from build123d import *

# Parameters (mm, degrees)
F1_DEPTH = 25.4
F3_D     = 7.874
F5_D     = 7.874


with BuildPart() as f1:
    # F0 (on Right) → F1 (new body, symmetric)
    with BuildSketch(Plane.YZ):
        with BuildLine():
            ThreePointArc((0, 160.2718698293), (0.8845331432, 155.615181848), (3.4149201504, 151.6071544741))
            Line((3.4149201504, 151.6071544741), (322.2393654787, -190.0440494609))
            ThreePointArc((322.2393654787, -190.0440494609), (323.4580585518, -191.9333664625), (323.9420015649, -194.1289371625))
            Line((323.9420015649, -194.1289371625), (327.3172136475, -280.67))
            Line((327.3172136475, -280.67), (336.2139723666, -280.67))
            Line((336.2139723666, -280.67), (332.7884473544, -192.8389043312))
            ThreePointArc((332.7884473544, -192.8389043312), (331.8205613281, -188.4477629311), (329.3831751819, -184.6691289279))
            Line((329.3831751819, -184.6691289279), (10.5974600752, 156.9405718319))
            ThreePointArc((10.5974600752, 156.9405718319), (9.3322665716, 158.9445855188), (8.89, 161.2729295095))
            Line((8.89, 161.2729295095), (8.89, 206.0665714286))
            Line((8.89, 206.0665714286), (0, 206.0665714286))
            Line((0, 206.0665714286), (0, 160.2718698293))
        make_face()
    extrude(amount=F1_DEPTH, both=True)

    # F3 (through all)
    with Locations(Plane(origin=(0, 8.89, 0), x_dir=(-1, 0, 0), z_dir=(0, 1, 0))):
        with Locations((0, 183.669750469)):
            Hole(F3_D / 2)

    # F5 (through all)
    with Locations(Plane(origin=(0, 315.8902243159, 12.3201225744), x_dir=(1, 0, 0), z_dir=(0, -0.9992403167, -0.0389716498))):
        with Locations((0, -227.6844431866), (0, -272.1344431866)):
            Hole(F5_D / 2)


solid = f1.part
Model file for the job. Use its own axes, mm. A direction names the side the tool comes from. Round coordinates to 2 decimals unless told otherwise and drop trailing zeros. Loops run counter-clockwise (first coordinate to the right, second up) from the corner with the lowest first, then second, coordinate; pieces in that order, holes last.
1. Drop flat-ended pins along their axis: P1, Ø2, axis at x = -19.5, y = 93.5, coming from the +Z side; P2, Ø4, axis at x = -4, z = -43.5, coming from the -Y side; P3, Ø10, axis at x = -3, z = -193.5, coming from the +Y side. Give the stop position or say it passes through.
Check values:
P1: stops at z = 69.17
P2: stops at y = 183.62
P3: stops at y = 333.01
2. Band-saw the part on B-B, the plane y = 33.5. List the corners of the cut face in (x, z).
Check values:
outline: (-25.4, 119.37) - (25.4, 119.37) - (25.4, 132.4) - (-25.4, 132.4) - close
3. Wall check: probe 1 along Z at (x, y) = (0, 3.5); probe 2 along Z at (x, y) = (0, 2); probe 3 along Y at (x, z) = (17, 79). Give the ranges that are in metal, low to high.
Check values:
probe 1: z = 151.52 to 179.73, 187.61 to 206.07
probe 2: z = 153.43 to 179.73, 187.61 to 206.07
probe 3: y = 71.17 to 83.33
4. Tool access for faces 1 (the flat face through (0.36, 160.6, -16.83)), 2 (the flat face through (0, 8.89, 188)): list every direction of +Z, -Z, +X, -X, +Y, -Y with a clear straight run to the whole face (end or side of a thin tool).
Check values:
face 1: -Z, +X, -X, -Y
face 2: +Z, +X, -X, +Y
5. Band-saw the part on A-A, the plane x = -18.5. List the corners of the cut face in (y, z), and give its area (3 significant figures).
Check values:
outline: (0, 160.27) arc R12.7 ccw to (3.41, 151.61) - (322.24, -190.04) arc R6.35 cw to (323.94, -194.13) - (327.32, -280.67) - (336.21, -280.67) - (332.79, -192.84) arc R12.7 ccw to (329.38, -184.67) - (10.6, 156.94) arc R6.35 cw to (8.89, 161.27) - (8.89, 206.07) - (0, 206.07) - close
area: 5,460 mm2
6. Band-saw the part on C-C, the plane z = -81.5. List the corners of the cut face in (x, y), and give its area (3 significant figures).
Check values:
outline: (-25.4, 220.95) - (25.4, 220.95) - (25.4, 233.11) - (-25.4, 233.11) - close
area: 618 mm2
